Part print with two shaded views. Sizes in mm from the minimum x, y, z corner. Round coordinates to 2 decimals unless told otherwise and drop trailing zeros. Order: outer loops, then holes, each group sorted by start corner. A loop starts at its lowest first (then second) coordinate and runs counter-clockwise, first axis right, second up. Notation, with made-up numbers: (-12.75, -2) - (0.25, -2) arc R19 ccw to (0.25, 14) - close; hole circle Ø6 at (76, -27). An arc over 180 degrees is marked (long way). Answer as CSV lines item,"result". Start each with the question number.
1. Wall check: line 1 along Y through (x, z) = (7.5, 1.2) (1 decimal); line 2 along Y through (x, z) = (19.5, 0.3); line 3 along X through (y, z) = (61.5, 0.3). Give the ranges that are in metal, low to high. Write a range as [from, to].
2. Band-saw the part on A-A on z = 0.3. List the corners of the cut face in (x, y).
3. Band-saw the part on D-D on y = 20.5. List the corners of the cut face in (x, z) (1 decimal).
4. Band-saw the part on B-B on y = 48.5. List the corners of the cut face in (x, z).
5. Band-saw the part on C-C on x = 21. List the corners of the cut face in (y, z) (1 decimal).
6. Pin check, flat tips, straight feed: pin 1 Ø0.8 at (y, z) = (2, 0.5) entering from +X; pin 2 Ø0.6 at (x, z) = (7.5, 0.5) entering from -Y. Stop position of each tip, or through.
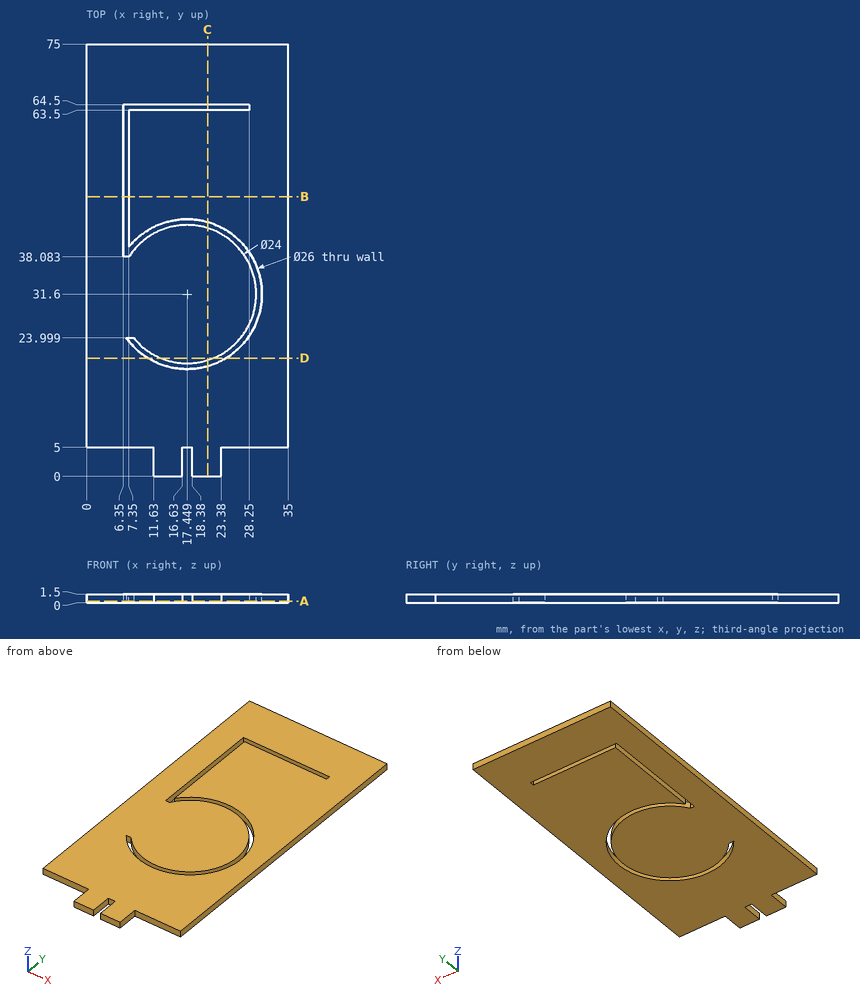
Reply:
1,line 1,"y = [5, 23.2], [24, 38.3], [40, 63.5], [64.5, 75]"
1,line 2,"y = [0, 18.76], [19.78, 43.42], [44.44, 63.5], [64.5, 75]"
1,line 3,"x = [0, 6.35], [7.35, 35]"
2,outline,"(0, 5) - (11.63, 5) - (11.63, 0) - (16.63, 0) - (16.63, 5) - (18.38, 5) - (18.38, 0) - (23.38, 0) - (23.38, 5) - (35, 5) - (35, 75) - (0, 75) - close; hole (6.35, 38.08) - (7.35, 38.08) arc R12 cw (long way) to (8.16, 24) - (6.9, 24) arc R13 ccw (long way) to (7.35, 39.79) - (7.35, 63.5) - (28.25, 63.5) - (28.25, 64.5) - (6.35, 64.5) - close"
3,outline,"(0, 0) - (10.7, 0) - (10.7, 1.5) - (0, 1.5) - close; (12.9, 0) - (22, 0) - (22, 1.5) - (12.9, 1.5) - close; (24.2, 0) - (35, 0) - (35, 1.5) - (24.2, 1.5) - close"
4,outline,"(0, 0) - (6.35, 0) - (6.35, 1.5) - (0, 1.5) - close; (7.35, 0) - (35, 0) - (35, 1.5) - (7.35, 1.5) - close"
5,outline,"(0, 0) - (19.1, 0) - (19.1, 1.5) - (0, 1.5) - close; (20.1, 0) - (43.1, 0) - (43.1, 1.5) - (20.1, 1.5) - close; (44.1, 0) - (63.5, 0) - (63.5, 1.5) - (44.1, 1.5) - close; (64.5, 0) - (75, 0) - (75, 1.5) - (64.5, 1.5) - close"
6,pin 1,"stops at x = 23.38"
6,pin 2,"stops at y = 5"
